Part model, mm, in its own coordinate system. Round coordinates to 2 decimals unless told otherwise and drop trailing zeros. Loops run counter-clockwise (first coordinate to the right, second up) from the corner with the lowest first, then second, coordinate; pieces in that order, holes last. Notation, with made-up numbers: (14.5, -21.75) -> (54.5, -21.75) arc R23 ccw to (54.5, -10.75) -> close; hole circle Ø11 at (12.5, 20). An arc over 180 degrees is marked (long way). Answer as CSV lines item,"result".
from build123d import *

# Parameters (mm, degrees)
SKETCH1_R               = 7.9375
SKETCH1_R_2             = 6.4643
BOSS_EXTRUDE1_DEPTH     = 299.825008041
CUT_EXTRUDE1_DEPTH      = 9.525
CUT_EXTRUDE1_DEPTH_BACK = 9.525


with BuildPart() as part:
    # Sketch1 → Boss-Extrude1 (new body)
    with BuildSketch(Plane(origin=(0, 0, 0), x_dir=(1, 0, 0), z_dir=(0, 1, 0))):
        with Locations(Location((0, 0, 0), (0, 0, 156.421821522))):
            Circle(SKETCH1_R)
        with Locations(Location((0, 0, 0), (0, 0, 150.583203301))):
            Circle(SKETCH1_R_2, mode=Mode.SUBTRACT)
    extrude(amount=BOSS_EXTRUDE1_DEPTH)

    # Sketch2 → Cut-Extrude1 (cut, two sides: drawn at the far end of the back side and taken through both)
    with BuildSketch(Plane(origin=(0, 0, 0), x_dir=(0, 0, -1), z_dir=(1, 0, 0)).offset(-CUT_EXTRUDE1_DEPTH_BACK)):
        with BuildLine():
            Line((3.175, 299.825008041), (3.175, 274.425008041))
            ThreePointArc((3.175, 274.425008041), (0, 271.250008041), (-3.175, 274.425008041))
            Line((-3.175, 274.425008041), (-3.175, 299.825008041))
            Line((-3.175, 299.825008041), (3.175, 299.825008041))
        make_face()
    extrude(amount=CUT_EXTRUDE1_DEPTH + CUT_EXTRUDE1_DEPTH_BACK, mode=Mode.SUBTRACT)


solid = part.part
Q1. Drop flat-ended pins along their axis: P1, Ø1.8, axis at x = -6.5, y = 292, coming from the +Z side; P2, Ø0.8, axis at x = 6.5, y = 281, coming from the +Z side; P3, Ø2, axis at y = 90.5, z = -5, coming from the -X side. Give the stop position or say it passes through.
Geometry results:
P1,"z = 5.63"
P2,"z = 5.08"
P3,"x = -6.86"
Q2. Saw through at B-B, the plane z = 0. Write the cut outline in (x, y), then the cut area to 3 significant figures.
Geometry results:
outline,"(-7.94, 0) -> (-6.46, 0) -> (-6.46, 271.25) -> (-7.94, 271.25) -> close; (6.46, 0) -> (7.94, 0) -> (7.94, 271.25) -> (6.46, 271.25) -> close"
area,"799 mm2"
Q3. Saw through at A-A, the plane x = 0. Write the cut outline in (y, z) (1 decimal), then the cut area to 3 significant figures.
Geometry results:
outline,"(0, -7.9) -> (299.8, -7.9) -> (299.8, -6.5) -> (0, -6.5) -> close; (0, 6.5) -> (299.8, 6.5) -> (299.8, 7.9) -> (0, 7.9) -> close"
area,"883 mm2"
Q4. Saw through at C-C, the plane y = 90.5. Write the cut outline in (x, z) (1 decimal).
Geometry results:
outline,"circle Ø15.9 at (0, 0); hole circle Ø12.9 at (0, 0)"
Q5. Two-plate mould, pull along Z, no slides. Class faces 1 (the face through (3.216, 147.814, 7.257)), 2 (the face through (6.4, 147.8, -0.9)), 3 (the face through (0, 299.825, -7)): pulls with the +Z half, pulls with the -Z half, needs draft (parallel to the pull), parting line crosses it, or undercut.
Geometry results:
face 1,"parting line crosses it"
face 2,"undercut"
face 3,"needs draft"
Q6. Drill centre lines: line 1 along Z through (x, y) = (0, 238.5); line 2 along Z through (x, y) = (-0.5, 54). Where is each one in solid material? Low to high.
Geometry results:
line 1,"-7.94 to -6.46, 6.46 to 7.94"
line 2,"-7.92 to -6.44, 6.44 to 7.92"
